```python
from build123d import *
from build123d.topology import SkipClean

# Parameters (mm, degrees)
SKETCH_1_W           = 20
SKETCH_1_H           = 60.00000000000001
SKETCH_1_R           = 1.7000000000000004
SKETCH_1_R_2         = 1.7
EXTRUDE_1_DEPTH      = 10
SKETCH_6_W           = 60.00000000000001
SKETCH_6_H           = 50.00000000000001
EXTRUDE_4_DEPTH      = 12
SKETCH_7_R           = 2.200000000000002
SKETCH_7_R_2         = 2.2
CUT_EXTRUDE_3_DEPTH  = 67.51315659326356
EXTRUDE_5_OUTLINE_R  = 2.2
EXTRUDE_5_DEPTH      = 5
CUT_EXTRUDE_7_DEPTH  = 5
SKETCH_14_R          = 2.2
CUT_EXTRUDE_8_DEPTH  = 5
CUT_EXTRUDE_START    = -17
CUT_EXTRUDE_9_DEPTH  = 17
SKETCH_18_W          = 6.800000000000008
SKETCH_18_H          = 2.000000000000014
SKETCH_18_W_2        = 6.799999999999994
SKETCH_18_H_2        = 2.0000000000000036
EXTRUDE_10_DEPTH     = 10
CUT_EXTRUDE_10_DEPTH = 62.35829229692095
CUT_EXTRUDE_11_DEPTH = 3.3
FILLET_1_R           = 5
FILLET_2_R           = 3


# Read off the part's stored shape, not the designer's step: 凸台-拉伸5
with BuildPart() as part:
    # 草图1 → 凸台-拉伸1 (new body)
    with BuildSketch(Plane(origin=(0, 0, 0), x_dir=(1, 0, 0), z_dir=(0, 1, 0))):
        Rectangle(SKETCH_1_W, SKETCH_1_H)
        with Locations(Location((-7.000000000000025, 5.2e-15, 0), (0, 0, 270))):
            Circle(SKETCH_1_R, mode=Mode.SUBTRACT)
        with Locations(Location((-2.429e-14, 5.2e-15, 0), (0, 0, 270))):
            Circle(SKETCH_1_R_2, mode=Mode.SUBTRACT)
        with Locations(Location((2.949e-14, 7.000000000000025, 0), (0, 0, 270))):
            Circle(SKETCH_1_R, mode=Mode.SUBTRACT)
        with Locations(Location((-4.48e-15, -7.000000000000048, 0), (0, 0, 270))):
            Circle(SKETCH_1_R, mode=Mode.SUBTRACT)
    extrude(amount=EXTRUDE_1_DEPTH)

    # 草图6 → 凸台-拉伸4 (add)
    with BuildSketch(Plane(origin=(10, 0, 0), x_dir=(0, 0, -1), z_dir=(1, 0, 0))):
        with Locations((0, 25.000000000000004)):
            Rectangle(SKETCH_6_W, SKETCH_6_H)
    extrude(amount=EXTRUDE_4_DEPTH)

    # 草图7 → 切除-拉伸3 (cut, through all)
    with BuildSketch(Plane(origin=(22, 0, 0), x_dir=(0, 0, -1), z_dir=(1, 0, 0))):
        with Locations((-22.500000000000014, 30)):
            Circle(SKETCH_7_R)
        with Locations((-22.500000000000014, 20)):
            Circle(SKETCH_7_R)
        Polygon((-18.20000000000001, 14.8), (22.199999999999985, 14.800000000000002), (22.199999999999985, 35.2), (-18.20000000000001, 35.2), align=None)
        with Locations((26.49999999999999, 30.000000000000007)):
            Circle(SKETCH_7_R)
        with Locations((26.49999999999999, 20.000000000000004)):
            Circle(SKETCH_7_R)
        Polygon((22.199999999999985, 26.00000000000001), (22.199999999999985, 23.999999999999996), (28.999999999999986, 24.000000000000004), (28.99999999999999, 26.00000000000001), align=None)
        Polygon((-25.000000000000014, 24), (-18.200000000000014, 24), (-18.20000000000001, 26.000000000000004), (-25.000000000000014, 26.000000000000004), align=None)
        with Locations((-5.159597133486693, 43.79385241571819)):
            Circle(SKETCH_7_R_2)
        with Locations((5.159597133486693, 43.79385241571819)):
            Circle(SKETCH_7_R_2)
    extrude(amount=-CUT_EXTRUDE_3_DEPTH, mode=Mode.SUBTRACT)

    # 凸台-拉伸5 outline → 凸台-拉伸5 (add)
    with SkipClean():  # the faces are left unmerged after this step: merging them gives an invalid solid
        with BuildSketch(Plane.ZY.offset(-10)):
            with BuildLine():
                Line((30, 10), (30, 35.4))
                Line((30, 35.4), (5.159597133, 48.793852416))
                Line((5.159597133, 48.793852416), (-5.159597133, 48.793852416))
                ThreePointArc((-5.159597133, 48.793852416), (-10.159597133, 43.793852416), (-5.159597133, 38.793852416))
                Line((-5.159597133, 38.793852416), (5, 38.793852416))
                Line((5, 38.793852416), (5, 10))
                Line((5, 10), (30, 10))
            make_face()
            with Locations((22.5, 20)):
                Circle(EXTRUDE_5_OUTLINE_R, mode=Mode.SUBTRACT)
            with Locations((-5.159597133, 43.793852416)):
                Circle(EXTRUDE_5_OUTLINE_R, mode=Mode.SUBTRACT)
            with Locations((5.159597133, 43.793852416)):
                Circle(EXTRUDE_5_OUTLINE_R, mode=Mode.SUBTRACT)
            with Locations((22.5, 30)):
                Circle(EXTRUDE_5_OUTLINE_R, mode=Mode.SUBTRACT)
        extrude(amount=EXTRUDE_5_DEPTH)

    # 草图13 → 切除-拉伸7 (cut)
    with BuildSketch(Plane.ZY.offset(-5)):
        with BuildLine():
            Line((26.400000000000016, 30), (26.400000000000016, 20))
            ThreePointArc((26.400000000000016, 20), (22.500000000000014, 16.099999999999998), (18.600000000000012, 20))
            Line((18.600000000000012, 20), (18.60000000000001, 30))
            ThreePointArc((18.60000000000001, 30), (22.500000000000014, 33.900000000000006), (26.400000000000016, 30))
        make_face()
    extrude(amount=-CUT_EXTRUDE_7_DEPTH, mode=Mode.SUBTRACT)

    # 草图14 → 切除-拉伸8 (cut)
    with BuildSketch(Plane(origin=(10, 0, 0), x_dir=(0, 0, -1), z_dir=(1, 0, 0))):
        with Locations((-11.800000000000018, 25)):
            Circle(SKETCH_14_R)
    extrude(amount=-CUT_EXTRUDE_8_DEPTH, mode=Mode.SUBTRACT)

    # 草图16 → 切除-拉伸9 (cut)
    with BuildSketch(Plane.ZY.offset(-5).offset(CUT_EXTRUDE_START)):
        with BuildLine():
            Line((5.159597133486693, 48.793852415718185), (30, 35.40000000000001))
            Line((30, 35.40000000000001), (30, 50))
            Line((30, 50), (-30, 50))
            Line((-30, 50), (-29.999999999999996, 35.2))
            Line((-29.999999999999996, 35.2), (-7.663336701878596, 48.121818239713186))
            ThreePointArc((-7.663336701878596, 48.121818239713186), (-6.455778231949604, 48.622922156360524), (-5.1595971334867095, 48.793852415718185))
            Line((-5.1595971334867095, 48.793852415718185), (5.159597133486693, 48.793852415718185))
        make_face()
    extrude(amount=CUT_EXTRUDE_9_DEPTH, mode=Mode.SUBTRACT)

    # 草图18 → 凸台-拉伸10 (add)
    with BuildSketch(Plane.ZY.offset(-10)):
        with Locations((-25.599999999999987, 25.000000000000004)):
            Rectangle(SKETCH_18_W, SKETCH_18_H)
        with Locations((21.60000000000001, 25)):
            Rectangle(SKETCH_18_W_2, SKETCH_18_H_2)
    extrude(amount=-EXTRUDE_10_DEPTH)

    # 草图19 → 切除-拉伸10 (cut, through all)
    with BuildSketch(Plane.XZ):
        with BuildLine():
            Line((-3.0000000000000244, 9.539392014169463), (-3.0000000000000244, 30))
            Line((-3.0000000000000244, 30), (-10, 30))
            Line((-10, 30), (-10, -1.2700383e-09))
            ThreePointArc((-10.000000000000028, -1.27003874e-09), (-8.06225774867426, 5.916079782587651), (-3.000000000000024, 9.539392014169465))
        make_face()
        with BuildLine():
            ThreePointArc((-3.0000000000000244, -9.539392014169461), (-8.062257747922892, -5.916079783611588), (-10.000000000000028, -1.27003874e-09))
            Line((-10, -1.2700383e-09), (-10, -30))
            Line((-10, -30), (-3.000000000000025, -30))
            Line((-3.0000000000000244, -30), (-3.0000000000000244, -9.539392014169465))
        make_face()
    extrude(amount=-CUT_EXTRUDE_10_DEPTH, mode=Mode.SUBTRACT)

    # 草图20 → 切除-拉伸11 (cut)
    with BuildSketch(Plane(origin=(10, 0, 0), x_dir=(0, 0, -1), z_dir=(1, 0, 0))):
        Polygon((-7.643078061834704, 24.999999999999993), (-9.721539030917363, 28.600000000000012), (-13.878460969082674, 28.600000000000012), (-15.956921938165337, 24.999999999999993), (-13.878460969082676, 21.399999999999984), (-9.721539030917361, 21.399999999999984), align=None)
    extrude(amount=-CUT_EXTRUDE_11_DEPTH, mode=Mode.SUBTRACT)

    # 圆角1
    fillet_1_edges = [part.edges().sort_by_distance(p)[0] for p in [
        (13.5, 35.400000000000006, 30),
        (16, 48.793852415718185, 5.159597133486693),
        (16, 35.2, -29.999999999999996),
        (-3.0000000000000244, 5, 30),
        (-3.000000000000024, 5, 9.539392014169465),
        (-3.000000000000025, 5, -30),
        (-3.000000000000025, 5, -9.539392014169465),
        (22, 0, 0),
    ]]
    fillet(fillet_1_edges, radius=FILLET_1_R)

    # 圆角2
    fillet_2_edges = [part.edges().sort_by_distance(p)[0] for p in [
        (7.5, 38.793852416, 5),
        (7.5, 10, 5),
    ]]
    fillet(fillet_2_edges, radius=FILLET_2_R)


solid = part.part
```
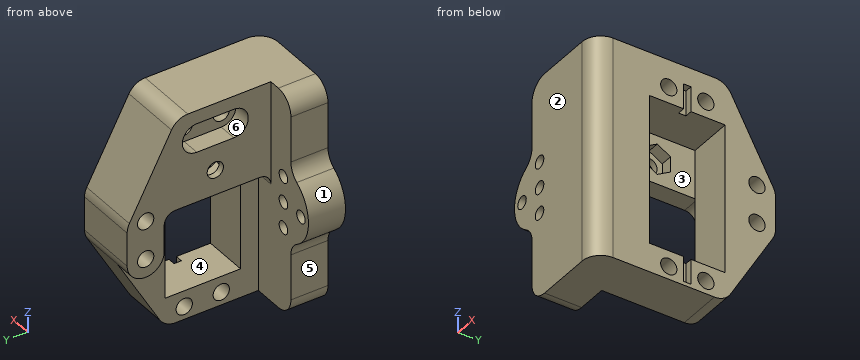
Geometry: final body of the model. Coordinates: model frame, mm. Face numbers are marked on the shaded views. A direction names the side the tool comes from. Round coordinates to 2 decimals unless told otherwise and drop trailing zeros. Write each loop counter-clockwise with the first axis right and the second up, starting at its lowest first coordinate (ties: lowest second). Pieces come first, ordered by that corner, then holes.
Item 1: Set-up query: the marked faces 4, 5 and 6. Return all of +Z, -Z, +X, -X, +Y, -Y with unobstructed straight access to the full face (end or side cutting, diameter ignored); none if empty.
Item 2: Section query B-B (y = 3). Return loops of the section in (x, z), plus the area to 3 significant figures.
Item 3: Pin query (flat end, axial travel): P1, Ø5, axis at y = 30, z = 22.5, coming from the -X side; P2, Ø1.6, axis at x = 21.5, z = 20.5, coming from the -Y side; P3, Ø3, axis at y = 40.5, z = 16.5, coming from the -X side. Return the tip coordinate at first contact, or that it passes through.
Item 4: Section query A-A (z = 0). Return loops of the section in (x, y), plus the area to 3 significant figures.
Item 5: Section query C-C (x = 0). Return loops of the section in (y, z), plus the area to 3 significant figures.
Item 6: Section query D-D (z = 22.5). Return loops of the section in (x, y).
Item 7: Mould query, pull axis Y, two halves, no side actions, for the marked faces 1, 2 and 3. Classes: +Y half, -Y half, draft (parallel to the pull), parting line (faces both ways), or undercut.
Item 8: Material intervals for L1, parallel to Y at x = 13.25, z = -26.5; L2, parallel to Y at x = 16.5, z = 2; L3, parallel to X at y = 27, z = 20.5, sorted ascending.
Completed:
1. face 4: +X, -X
1. face 5: -Z, -X, +Y, -Y
1. face 6: -X
2. outline: (-5.33, -8.46) arc R5 cw to (-3, -12.69) - (-3, -25) arc R5 ccw to (2, -30) - (21.58, -30) - (21.58, 30) - (2, 30) arc R5 ccw to (-3, 25) - (-3, 12.69) arc R5 cw to (-5.33, 8.46) arc R10 ccw to start; hole circle Ø3.4 at (-7, 0); hole circle Ø3.4 at (0, -7); hole circle Ø3.4 at (0, 0); hole circle Ø3.4 at (0, 7)
2. area: 1,530 mm2
3. P1: stops at x = 10
3. P2: stops at y = 1.64
3. P3: stops at x = 5
4. outline: (-10, 0) - (-8.7, 0) - (-8.7, 10) - (-10, 10) - close; (-5.3, 0) - (-1.7, 0) - (-1.7, 10) - (-5.3, 10) - close; (1.7, 0) - (17, 0) arc R5 ccw to (22, 5) - (22, 14.8) - (10, 14.8) - (10, 10) - (1.7, 10) - close; (5, 38.79) - (10, 38.79) - (10, 35.2) - (22, 35.2) - (22, 48.79) - (5, 48.79) - close
4. area: 517 mm2
5. outline: (0, -29.58) - (10, -29.58) - (10, -8.7) - (0, -8.7) - close; (0, -5.3) - (10, -5.3) - (10, -1.7) - (0, -1.7) - close; (0, 1.7) - (10, 1.7) - (10, 5.3) - (0, 5.3) - close; (0, 8.7) - (10, 8.7) - (10, 29.58) - (0, 29.58) - close
5. area: 490 mm2
6. outline: (-3, 0) - (17, 0) arc R5 ccw to (22, 5) - (22, 17.8) - (10, 17.8) - (10, 16.1) - (5, 16.1) - (5, 10) - (-3, 10) - close; (5, 33.9) - (10, 33.9) - (10, 32.2) - (22, 32.2) - (22, 39.44) - (5, 39.44) - close; (10, 22.2) - (22, 22.2) - (22, 24) - (20, 24) - (20, 26) - (22, 26) - (22, 27.8) - (10, 27.8) - close
7. face 1: draft
7. face 2: -Y half
7. face 3: undercut
8. L1: y = 0 to 17.8, 22.2 to 27.8, 32.2 to 37.22
8. L2: y = 0 to 14.8, 35.2 to 48.79
8. L3: x = 10 to 22
